Read the model definition and answer for the solid it produces. Units are mm, in the model's axes. Coordinates: 2 decimals unless noted, no trailing zeros. Loops run counter-clockwise (first coordinate to the right, second up) from the corner with the lowest first, then second, coordinate; pieces in that order, holes last. Notation, with made-up numbers: (36.25, -15) - (95.25, -15) arc R25 cw to (95.25, 23) - close; hole circle Ø10 at (-37.5, -31.75). An arc over 180 degrees is marked (long way). Use CSV: the item, a comma, the result in double quotes.
```python
from build123d import *

# Parameters (mm, degrees)
SKETCH2_W            = 106
SKETCH2_H            = 106
BOSS_EXTRUDE3_DEPTH  = 5
SKETCH3_W            = 103
SKETCH3_H            = 103
CUT_EXTRUDE1_DEPTH   = 3
SKETCH4_W            = 9
SKETCH4_H            = 3.784346923
CUT_EXTRUDE2_DEPTH   = 10
FILLET1_R            = 3
SKETCH5_W            = 28
SKETCH5_H            = 101
CUT_EXTRUDE3_DEPTH   = 10
CUT_EXTRUDE5_DEPTH   = 2
LPATTERN1_COUNT      = 4
LPATTERN1_PITCH      = 22
LPATTERN1_COUNT_DIR2 = 3
LPATTERN1_PITCH_DIR2 = 20


with BuildPart() as part:
    # Sketch2 → Boss-Extrude3 (new body)
    with BuildSketch(Plane(origin=(0, 0, 0), x_dir=(1, 0, 0), z_dir=(0, 1, 0))):
        with Locations((48.527443435, -44.155148704)):
            Rectangle(SKETCH2_W, SKETCH2_H)
    extrude(amount=BOSS_EXTRUDE3_DEPTH)

    # Sketch3 → Cut-Extrude1 (cut)
    with BuildSketch(Plane(origin=(0, 0, 0), x_dir=(1, 0, 0), z_dir=(0, 1, 0))):
        with Locations((48.527443435, -44.155148704)):
            Rectangle(SKETCH3_W, SKETCH3_H)
    extrude(amount=CUT_EXTRUDE1_DEPTH, mode=Mode.SUBTRACT)

    # Sketch4 → Cut-Extrude2 (cut)
    with BuildSketch(Plane.XY.offset(97.155148704)):
        with Locations((83.877443435, 1.892173462)):
            Rectangle(SKETCH4_W, SKETCH4_H)
    extrude(amount=-CUT_EXTRUDE2_DEPTH, mode=Mode.SUBTRACT)

    # Fillet1
    # the kernel refuses this fillet: 3 mm, written as the material it takes off along each edge
    with BuildSketch(Plane(origin=(101.527443435, 5, -16.344851296), x_dir=(0, -1, 0), z_dir=(0, 0, 1)), Plane(origin=(-11.972556565, 5, -8.844851296), x_dir=(0, -1, 0), z_dir=(1, 0, 0)), Plane(origin=(-4.472556565, 5, 104.655148704), x_dir=(0, -1, 0), z_dir=(0, 0, -1))) as fillet1_piece_1:
        with BuildLine():
            CenterArc((FILLET1_R, -FILLET1_R), FILLET1_R, 90, 90)
            Line((0, -FILLET1_R), (0, 0))
            Line((0, 0), (FILLET1_R, 0))
        make_face()
    extrude(amount=121, mode=Mode.SUBTRACT)
    with BuildSketch(Plane(origin=(109.027443435, 5, 97.155148704), x_dir=(0, 0, -1), z_dir=(-1, 0, 0))) as fillet1_piece_2:
        with BuildLine():
            CenterArc((FILLET1_R, FILLET1_R), FILLET1_R, 180, 90)
            Line((0, FILLET1_R), (0, 0))
            Line((0, 0), (FILLET1_R, 0))
        make_face()
    extrude(amount=121, mode=Mode.SUBTRACT)

    # Sketch5 → Cut-Extrude3 (cut)
    with BuildSketch(Plane(origin=(0, 5, 0), x_dir=(1, 0, 0), z_dir=(0, 1, 0))):
        with Locations((83.527443435, -44.655148704)):
            Rectangle(SKETCH5_W, SKETCH5_H)
    extrude(amount=-CUT_EXTRUDE3_DEPTH, mode=Mode.SUBTRACT)

    # Sketch6 → Cut-Extrude5 (cut)
    with BuildSketch(Plane(origin=(0, 5, 0), x_dir=(1, 0, 0), z_dir=(0, 1, 0))):
        Polygon((49.377443435, -69.405148704), (49.377443435, -85.405148704), (65.377443435, -85.405148704), (65.377443435, -69.405148704), (65.377443435, -64.405148704), (49.377443435, -64.405148704), align=None)
    cut_extrude5 = extrude(amount=-CUT_EXTRUDE5_DEPTH, mode=Mode.SUBTRACT)

    # LPattern1: Cut-Extrude5 4 × 3
    with Locations(*[(-j * LPATTERN1_PITCH_DIR2, 0, -i * LPATTERN1_PITCH) for i in range(LPATTERN1_COUNT) for j in range(LPATTERN1_COUNT_DIR2) if (i, j) != (0, 0)]):
        add(cut_extrude5, mode=Mode.SUBTRACT)


solid = part.part
```
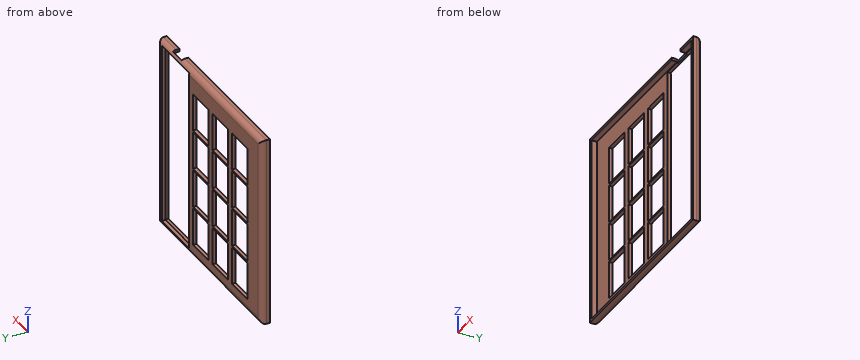
Q1. The part is cut by section B-B on z = 11. Determine the outline of the cut face in (x, y), and give its area (3 significant figures).
Reported:
outline,"(-4.47, 0) - (-2.97, 0) - (-2.97, 3) - (9.38, 3) - (9.38, 5) - (-1.47, 5) arc R3 ccw to (-4.47, 2) - close; (25.38, 3) - (29.38, 3) - (29.38, 5) - (25.38, 5) - close; (45.38, 3) - (49.38, 3) - (49.38, 5) - (45.38, 5) - close; (65.38, 3) - (69.53, 3) - (69.53, 5) - (65.38, 5) - close; (97.53, 3) - (100.03, 3) - (100.03, 0) - (101.53, 0) - (101.53, 2) arc R3 ccw to (98.53, 5) - (97.53, 5) - close"
area,"65.1 mm²"
Q2. The part is cut by section C-C on x = 4. Determine the outline of the cut face in (y, z), and give its area (3 significant figures).
Reported:
outline,"(0, -8.84) - (2, -8.84) arc R3 ccw to (5, -5.84) - (5, 94.16) arc R3 ccw to (2, 97.16) - (0, 97.16) - (0, 95.66) - (3, 95.66) - (3, -7.34) - (0, -7.34) - close"
area,"217 mm²"
Q3. The part is cut by section A-A on x = 92.5. Determine the outline of the cut face in (y, z).
Reported:
outline,"(0, -8.84) - (2, -8.84) arc R3 ccw to (5, -5.84) - (3, -5.84) - (3, -7.34) - (0, -7.34) - close; (0, 95.66) - (3, 95.66) - (3, 95.16) - (4.83, 95.16) arc R3 ccw to (2, 97.16) - (0, 97.16) - close"
Q4. Given P1, Ø2, axis at y = 4, z = 56, coming from the -X side; P2, Ø1, axis at x = 53.5, y = 4, coming from the +Z side; P3, Ø2, axis at x = 54, y = 3.5, coming from the -Z side; P4, Ø3, axis at y = 3.5, z = 80, coming from the +X side, each flat-ended and moving along its own axis, determine where each tip first touches the part or whether it passes through.
Reported:
P1,"stops at x = -4.3"
P2,"stops at z = 96.75"
P3,"stops at z = -8.8"
P4,"stops at x = 101.53"
Q5. Find the intervals of material crossed by probe 1 along X at (y, z) = (1.8, 27); probe 2 along Z at (x, y) = (94, 2.25); probe 3 along X at (y, z) = (4.35, 58.5), in increasing order. Write a range as [from, to].
Reported:
probe 1,"x = [-4.47, -2.97], [100.03, 101.53]"
probe 2,"z = [-8.83, -7.34], [95.66, 97.14]"
probe 3,"x = [-3.34, 9.38], [25.38, 29.38], [45.38, 49.38], [65.38, 69.53], [97.53, 100.39]"
